Design review of the part built by this model. Coordinates are the model's own, in mm. Coordinates: 2 decimals unless noted, no trailing zeros. Loops run counter-clockwise (first coordinate to the right, second up) from the corner with the lowest first, then second, coordinate; pieces in that order, holes last. Notation, with made-up numbers: (38, -13.75) -> (52, -13.75) arc R12 ccw to (52, 6.25) -> close; hole circle Ø9 at (74.5, 83). An arc over 180 degrees is marked (long way). Answer as a JSON object with one key per item and string values.
```python
from build123d import *

# Parameters (mm, degrees)
BOSS_EXTRUDE1_DEPTH = 542.544
FILLET1_R           = 3.81


with BuildPart() as part:
    # Sketch1 → Boss-Extrude1 (new body)
    with BuildSketch(Plane.XY):
        Polygon((0, 4.68249), (0, -4.68249), (48.14824, 0), align=None)
    extrude(amount=BOSS_EXTRUDE1_DEPTH)

    # Fillet1
    fillet1_edges = [part.edges().sort_by_distance(p)[0] for p in [
        (0, -4.68249, 271.272),
        (0, 4.68249, 271.272),
    ]]
    fillet(fillet1_edges, radius=FILLET1_R)


solid = part.part
```
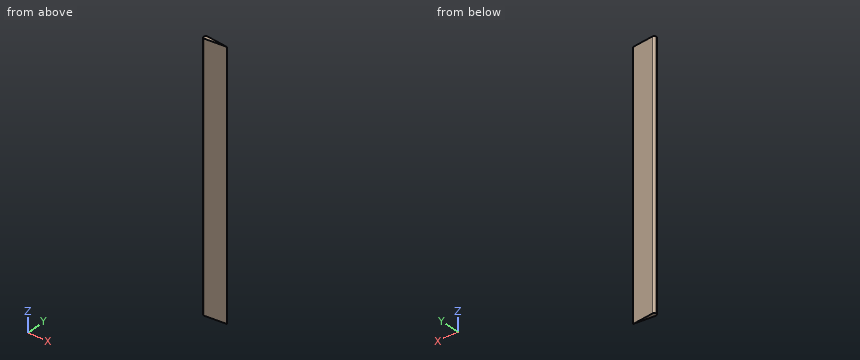
1) Wall thickness on probe 1 along Y at (x, z) = (43.5, 85); probe 2 along Y at (x, z) = (24.5, 473.5): over which ranges is each line inside the solid? List them lowest first.
Completed:
{"probe 1": "-0.45 to 0.45", "probe 2": "-2.3 to 2.3"}
2) Add section A-A, the plane z = 242. Give the boundary of the cut face in (x, y), and give its area (3 significant figures).
Completed:
{"outline": "(0, -0.48) arc R3.81 ccw to (4.18, -4.28) -> (48.15, 0) -> (4.18, 4.28) arc R3.81 ccw to (0, 0.48) -> close", "area": "218 mm²"}
3) Clearance check with flat-ended pins moving along their axes: pin 1 Ø3 at (x, z) = (13.5, 214.5) entering from +Y; pin 2 Ø5 at (x, z) = (17, 186) entering from +Y; pin 3 Ø1.5 at (x, z) = (18, 68) entering from -Y. State where each tip first meets the part, or that it passes through.
Completed:
{"pin 1": "y = 3.52", "pin 2": "y = 3.27", "pin 3": "y = -3"}
4) Add section C-C, the plane y = -2. Give the boundary of the cut face in (x, z), and give its area (3 significant figures).
Completed:
{"outline": "(0.31, 0) -> (27.58, 0) -> (27.58, 542.54) -> (0.31, 542.54) -> close", "area": "14,800 mm²"}
5) Add section B-B, the plane x = 30.5. Give the boundary of the cut face in (y, z).
Completed:
{"outline": "(-1.72, 0) -> (1.72, 0) -> (1.72, 542.54) -> (-1.72, 542.54) -> close"}
